For this review, take the finished solid that the model builds, in its own axes (mm). Face numbers are marked on the shaded views. A direction names the side the tool comes from. Give positions to 0.01 mm unless a question says otherwise; leave off trailing zeros. Loops run counter-clockwise (first coordinate to the right, second up) from the corner with the lowest first, then second, coordinate; pieces in that order, holes last.
Autodesk Inventor part; units mm, degrees
ref_plane "YZ Plane" through (0, 0, 0) normal (1, 0, 0) x (0, 1, 0)
ref_plane "XZ Plane" through (0, 0, 0) normal (0, 1, 0) x (-1, 0, 0)
ref_plane "XY Plane" through (0, 0, 0) normal (0, 0, 1) x (1, 0, 0)
sketch "Main Outline" plane through (0, 0, 0) normal (0, 0, 1) x (1, 0, 0)
  line L0 (0, 0) -> (304.8, 0) construction
  line L1 (304.8, 0) -> (304.8, 50.8) construction
  line L2 (304.8, 50.8) -> (0, 50.8) construction
  line L3 (0, 50.8) -> (0, 0) construction
  line L4 (0, 50.8) -> (0, 53.34) construction
  line L5 (0, 53.34) -> (304.8, 53.34) construction
  line L6 (304.8, 53.34) -> (304.8, 50.8) construction
  circle A0 centre (152.4, 23.8125) radius 17.4625 construction
  line L7 (152.4, 23.8125) -> (152.4, 0) construction
  circle A1 centre (152.4, 23.8125) radius 27.94 construction
  circle A2 centre (152.4, 23.8125) radius 21.59 construction
  line L8 (152.4, 23.8125) -> (144.1569, 60.2292) construction
  circle A3 centre (144.1569, 60.2292) radius 15.24 construction
  circle A4 centre (144.1569, 60.2292) radius 8.89 construction
  circle A5 centre (144.1569, 60.2292) radius 14.2875 construction
  arc A6 (163.8162, 72.0089) -> (128.198, 43.7805) centre (144.1569, 60.2292) ccw construction
  circle A7 centre (98.8106, 85.598) radius 32.258 construction
  circle A8 centre (124.5097, 147.0273) radius 32.258 construction
  circle A9 centre (174.158, 102.6533) radius 32.258 construction
  circle A10 centre (144.1569, 60.2292) radius 11.1125 construction
  circle A11 centre (152.4, 23.8125) radius 49.53 construction
  line L9 (144.1569, 60.2292) -> (124.5097, 147.0273) construction
  line L10 (144.1569, 60.2292) -> (98.8106, 85.598) construction
  line L11 (98.8106, 85.598) -> (174.158, 102.6533) construction
  line L12 (174.158, 102.6533) -> (144.1569, 60.2292) construction
  circle A12 centre (98.8106, 85.598) radius 9.5493 construction
  arc A13 (172.0498, 111.9669) -> (183.1109, 99.3313) centre (174.158, 102.6533) ccw construction
  circle A14 centre (124.5097, 147.0273) radius 9.5493 construction
  line L13 (96.7024, 94.9117) -> (172.0498, 111.9669) construction
  line L14 (183.1109, 99.3313) -> (165.6438, 52.2565) construction
  line L15 (92.161, 78.7444) -> (128.198, 43.7805) construction
  line L16 (172.0498, 111.9669) -> (174.158, 102.6533) construction
  line L17 (174.158, 102.6533) -> (183.1109, 99.3313) construction
  arc A15 (183.1109, 99.3313) -> (172.0498, 111.9669) centre (174.158, 102.6533) ccw construction
  arc A16 (165.6438, 52.2565) -> (163.8162, 72.0089) centre (144.1569, 60.2292) ccw construction
  arc A17 (128.198, 43.7805) -> (165.6438, 52.2565) centre (144.1569, 60.2292) ccw construction
  circle A18 centre (124.4396, 147.337) radius 32.258 construction
  circle A19 centre (124.3695, 147.6466) radius 32.258 construction
  circle A20 centre (124.2994, 147.9563) radius 32.258 construction
  line L18 (124.5097, 147.0273) -> (124.2994, 147.9563) construction
  circle A21 centre (124.5798, 146.7176) radius 32.258 construction
  circle A22 centre (117.4622, 43.2997) radius 9.525 construction
  circle A23 centre (175.54, 56.4459) radius 9.525 construction
  line L19 (152.4, 23.8125) -> (117.4622, 43.2997) construction
  line L20 (152.4, 23.8125) -> (175.54, 56.4459) construction
  line L21 (117.4622, 43.2997) -> (98.8106, 85.598) construction
  line L22 (175.54, 56.4459) -> (174.158, 102.6533) construction
  circle A24 centre (133.7342, 106.2753) radius 7.9375 construction
  line L23 (133.401, 150.5107) -> (165.496, 68.5894) construction
  circle A25 centre (152.4, 23.8125) radius 29.845 construction
  line L24 (114.985, 146.3422) -> (121.2977, 58.5849) construction
  circle A26 centre (99.0876, 85.443) radius 32.258 construction
  circle A27 centre (97.9793, 86.063) radius 32.258 construction
  line L25 (97.9793, 86.063) -> (98.8106, 85.598) construction
  circle A28 centre (98.2564, 85.908) radius 32.258 construction
  circle A29 centre (98.5335, 85.753) radius 32.258 construction
  circle A30 centre (152.4, 23.8125) radius 29.845 construction
  circle A31 centre (122.555, 23.8125) radius 6.35 construction
  circle A32 centre (179.3358, 36.6651) radius 6.35 construction
  line L26 (122.555, 23.8125) -> (152.4, 23.8125) construction
  line L27 (152.4, 23.8125) -> (182.245, 23.8125) construction
  circle A33 centre (182.245, 23.8125) radius 6.35 construction
  circle A34 centre (125.4642, 10.9599) radius 6.35 construction
  circle A35 centre (150.1885, 33.5827) radius 39.8623 construction
  line L28 (72.8944, 65.7819) -> (119.1902, 8.5205) construction
  circle A36 centre (174.708, 103.431) radius 32.258 construction
  line L29 (174.158, 102.6533) -> (174.708, 103.431) construction
  circle A37 centre (174.5246, 103.1717) radius 32.258 construction
  circle A38 centre (174.3413, 102.9125) radius 32.258 construction
  circle A39 centre (173.9747, 102.394) radius 32.258 construction
  line L30 (188.958, 24.3128) -> (206.0816, 95.9295) construction
  circle A40 centre (133.7342, 106.2753) radius 8.1693 construction
  arc A41 (85.4541, 115.7901) -> (94.2274, 135.7949) centre (79.2901, 130.4196) ccw construction
  arc A42 (156.6774, 149.9308) -> (173.2104, 135.6542) centre (172.4734, 151.5121) ccw construction
  line L31 (124.2994, 147.9563) -> (124.8602, 145.479) construction
  line L32 (114.3901, 145.7133) -> (114.9509, 143.236) construction
  line L33 (134.7695, 147.722) -> (134.2088, 150.1993) construction
  arc A43 (134.2088, 150.1993) -> (114.3901, 145.7133) centre (124.2994, 147.9563) ccw construction
  arc A44 (114.9509, 143.236) -> (134.7695, 147.722) centre (124.8602, 145.479) ccw construction
  line L34 (174.708, 103.431) -> (173.2414, 101.3571) construction
  line L35 (166.4126, 109.2972) -> (164.9461, 107.2234) construction
  line L36 (181.5368, 95.4909) -> (183.0033, 97.5647) construction
  arc A45 (183.0033, 97.5647) -> (166.4126, 109.2972) centre (174.708, 103.431) ccw construction
  arc A46 (164.9461, 107.2234) -> (181.5368, 95.4909) centre (173.2414, 101.3571) ccw construction
  line L37 (97.9793, 86.063) -> (100.196, 84.8229) construction
  line L38 (93.0188, 77.1963) -> (95.2355, 75.9562) construction
  line L39 (105.1564, 93.6897) -> (102.9398, 94.9298) construction
  arc A47 (102.9398, 94.9298) -> (93.0188, 77.1963) centre (97.9793, 86.063) ccw construction
  arc A48 (95.2355, 75.9562) -> (105.1564, 93.6897) centre (100.196, 84.8229) ccw construction
  circle A49 centre (117.4622, 43.2997) radius 3.9687 construction
  circle A50 centre (175.54, 56.4459) radius 3.9687 construction
  line L40 (152.4, 23.8125) -> (158.9889, -5.2961) construction
  arc A51 (89.3511, 54.6895) -> (85.9237, 49.6664) centre (88.3927, 51.6626) ccw construction
  arc A52 (201.2624, 75.7739) -> (196.006, 78.8314) centre (198.1744, 76.5122) ccw construction
  circle A53 centre (152.4, 23.8125) radius 14.224 construction
  circle A54 centre (133.7342, 106.2753) radius 3.9687 construction
  circle A55 centre (156.886, 3.9939) radius 6.35 construction
  circle A56 centre (156.886, 3.9939) radius 2.0828 construction
  circle A57 centre (152.4, 23.8125) radius 20.32 construction
  line L41 (132.9935, 29.8368) -> (152.4, 23.8125) construction
  line L42 (152.4, 23.8125) -> (167.3204, 37.6068) construction
  circle A58 centre (167.3204, 37.6068) radius 2.0828 construction
  circle A59 centre (167.3204, 37.6068) radius 3.9687 construction
  circle A60 centre (132.9935, 29.8368) radius 2.0828 construction
  circle A61 centre (132.9935, 29.8368) radius 3.9688 construction
  point P0 (173.9747, 102.394)
  point P1 (99.0876, 85.443)
  dimension "d18" = 99.06
  dimension "d58" = 64.516
  dimension "d86" = 64.516
  dimension "d0" = 304.8
  dimension "d1" = 50.8
  dimension "d2" = 2.54
  dimension "d3" = 34.925
  dimension "d4" = 23.8125
  dimension "d5" = 152.4
  dimension "d6" = 55.88
  dimension "d7" = 43.18
  dimension "d8" = 37.338
  dimension "d10" = 30.48
  dimension "d11" = 17.78
  dimension "d12" = 28.575
  dimension "d13" = 45.8366
  dimension "d14" = 64.516
  dimension "d15" = 64.516
  dimension "d16" = 64.516
  dimension "d17" = 22.225
  dimension "d19" = 51.9602
  dimension "d20" = 88.9939
  dimension "d21" = 19.0986
  dimension "d22" = 19.0986
  dimension "d23" = 19.0986
  dimension "d30" = 123.112
  dimension "d40" = 64.516
  dimension "d41" = 64.516
  dimension "d42" = 64.516
  dimension "d43" = 0.9525
  dimension "d44" = 0.3175
  dimension "d45" = 0.635
  dimension "d46" = 64.516
  dimension "d47" = 0.3175
  dimension "d48" = 19.05
  dimension "d49" = 19.05
  dimension "d50" = 40.005
  dimension "d51" = 40.005
  dimension "d52" = 46.228
  dimension "d54" = 46.228
  dimension "d55" = 15.875
  dimension "d56" = 41.4655
  dimension "d57" = 59.69
  dimension "d59" = 64.516
  dimension "d60" = 64.516
  dimension "d61" = 64.516
  dimension "d62" = 0.3175
  dimension "d63" = 0.3175
  dimension "d64" = 0.635
  dimension "d65" = 0.9525
  dimension "d73" = 12.7
  dimension "d74" = 12.7
  dimension "d76" = 59.69
  dimension "d78" = 12.7
  dimension "d79" = 12.7
  dimension "d80" = 64.516
  dimension "d81" = 0.9525
  dimension "d82" = 64.516
  dimension "d83" = 64.516
  dimension "d84" = 0.3175
  dimension "d85" = 0.635
  dimension "d88" = 0.3175
  dimension "d89" = 31.75
  dimension "d90" = 31.75
  dimension "d94" = 1.5875
  dimension "d95" = 20.32
  dimension "d96" = 1.5875
sketch "Upper CIM C-C Check" plane through (0, 0, 0) normal (0, 0, 1) x (1, 0, 0)
  arc A0 (3.4429, -22.6582) -> (3.4429, 22.6582) centre (0, 0) ccw construction
  arc A1 (90.4285, 9.4409) -> (90.4285, -9.4409) centre (88.9939, 0) ccw construction
  line L0 (88.9939, 0) -> (0, 0) construction
  line L1 (90.4285, 9.4409) -> (3.4429, 22.6582)
  line L2 (3.4429, -22.6582) -> (90.4285, -9.4409)
  arc A2 (90.4285, -9.4409) -> (90.4285, 9.4409) centre (88.9939, 0) ccw
  arc A3 (3.4429, 22.6582) -> (3.4429, -22.6582) centre (0, 0) ccw
  dimension "d24" = 45.8366
  dimension "d25" = 19.0986
  dimension "d26" = 78.9119
  dimension "d27" = 87.984
  dimension "d28" = 27.12
  dimension "d29" = 88.9939
sketch "Sketch3" plane through (0, 0, 0) normal (1, 0, 0) x (0, 1, 0)
  line L0 (0, 0) -> (50.8, 0)
  line L1 (50.8, 0) -> (50.8, -50.8)
  line L2 (50.8, -50.8) -> (0, -50.8)
  line L3 (0, -50.8) -> (0, 0)
  line L4 (3.175, -3.175) -> (47.625, -3.175)
  line L5 (47.625, -3.175) -> (47.625, -47.625)
  line L6 (47.625, -47.625) -> (3.175, -47.625)
  line L7 (3.175, -47.625) -> (3.175, -3.175)
  dimension "d115" = 50.8
  dimension "d116" = 50.8
  dimension "d117" = 44.45
  dimension "d118" = 44.45
  dimension "d119" = 3.175
  dimension "d120" = 3.175
extrude "Extrusion1" add sketch "Sketch3" along normal blind 304.8
sketch "Sketch4" plane through (0, 0, 0) normal (0, 0, 1) x (1, 0, 0)
  circle A0 centre (152.4, 23.8125) radius 9.525
  circle A1 centre (117.4622, 43.2997) radius 4.7625
  circle A2 centre (144.1569, 60.2292) radius 12.7
  point P0 (0, 0)
  point P1 (122.555, 23.8125)
  point P2 (125.4642, 10.9599)
  point P3 (182.245, 23.8125)
  point P4 (179.3358, 36.6651)
  dimension "d123" = 19.05
  dimension "d124" = 9.525
  dimension "d134" = 25.4
extrude "Extrusion2" cut sketch "Sketch4" against normal up to surface (3.175 mm away) contours A0 | A1
hole "Hole1" at (122.555, 23.8125, 0) at (182.245, 23.8125, 0) direction (0, 0, -1) diameter 6.5278 end up to surface
extrude "Extrusion3" cut sketch "Sketch4" against normal up to surface (50.8 mm away) contours A2
fillet "Fillet1" radius 25.4 2 edges at (135.6493, 50.8, -25.4) (152.6645, 50.8, -25.4)
equation "\"d3\" = r10"
equation "\"d6\" = g44"
equation "\"d7\" = g34"
equation "\"d10\" = g24"
equation "\"d11\" = g14"
equation "\"d12\" = r8"
equation "\"d13\" = p48"
equation "\"d14\" = cim"
equation "\"d15\" = cim"
equation "\"d16\" = cim"
equation "\"d17\" = r6"
equation "\"d21\" = p20"
equation "\"d22\" = p20"
equation "\"d23\" = p20"
equation "\"d24\" = p48"
equation "\"d25\" = p20"
equation "\"d29\" = d20"
equation "\"g14\" = 17.78"
equation "\"g24\" = 30.48"
equation "\"g34\" = 43.18"
equation "\"g44\" = 55.88"
equation "\"p20\" = 19.09859"
equation "\"p48\" = 45.83662"
equation "\"r10\" = 34.925"
equation "\"r9\" = 31.75"
equation "\"r8\" = 28.575"
equation "\"r7\" = 25.4"
equation "\"r6\" = 22.225"
equation "\"r5\" = 19.05"
equation "\"r4\" = 15.875"
equation "\"r3\" = 12.7"
equation "\"cim\" = 64.516"
equation "\"act\" = 28.448"
equation "\"actL\" = 23.749"
equation "\"UpperCimCCCheck\" = 2 * d27 + d26 + d28"
equation "\"LowerBeltPathCCCheck\" = 267"
properties material "Aluminum 6061"
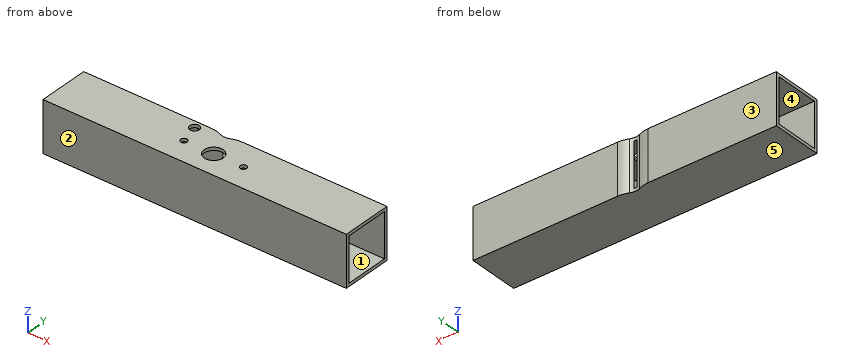
Item 1: Take a section at C-C on y = 11. Give the boundary of the cut face in (x, z) (3 decimals).
Answer:
outline: (0, -50.8) - (304.8, -50.8) - (304.8, -47.625) - (0, -47.625) - close; (0, -3.175) - (304.8, -3.175) - (304.8, 0) - (0, 0) - close
Item 2: Take a section at B-B on z = -33.5. Give the boundary of the cut face in (x, y) (3 decimals).
Answer:
outline: (0, 0) - (304.8, 0) - (304.8, 3.175) - (0, 3.175) - close; (0, 47.625) - (142.6, 47.625) arc R12.7 cw to (139.009, 48.619) arc R25.4 ccw to (128.712, 50.8) - (0, 50.8) - close; (145.714, 47.625) - (304.8, 47.625) - (304.8, 50.8) - (159.602, 50.8) arc R25.4 ccw to (149.305, 48.619) arc R12.7 cw to start
Item 3: For L1, parallel to Z at x = 187, y = 42 (3 decimals); L2, parallel to Y at x = 178, z = -25 (3 decimals); L3, parallel to Y at x = 155, z = -25 (3 decimals), list the stretches that pass through material, from the lowest coordinate up.
Answer:
L1: z = -50.8 to -47.625, -3.175 to 0
L2: y = 0 to 3.175, 47.625 to 50.8
L3: y = 0 to 3.175, 47.625 to 50.38
Item 4: Clearance check with flat-ended pins moving along their axes: pin 1 Ø5 at (y, z) = (44.5, -16.5) entering from +X; pin 2 Ø6 at (x, z) = (154, -35) entering from +Y; pin 3 Ø5 at (x, y) = (122.56, 23.81) entering from +Z (3 decimals). State where each tip first meets the part, or that it passes through.
Answer:
pin 1: passes through
pin 2: stops at y = 50.67
pin 3: stops at z = -47.625
Item 5: Take a section at D-D on x = 152.4. Give the boundary of the cut face in (y, z) (1 decimal), and give its area (3 significant figures).
Answer:
outline: (0, -50.8) - (49.8, -50.8) - (49.8, 0) - (33.3, 0) - (33.3, -3.2) - (47.6, -3.2) - (47.6, -47.6) - (3.2, -47.6) - (3.2, -3.2) - (14.3, -3.2) - (14.3, 0) - (0, 0) - close
area: 491 mm2
Item 6: The part is to be moulded in two halves that separate along Y. For the marked faces 3, 4 and 5, say which applies: released by +Y, released by -Y, zero draft, split by the parting line, or undercut.
Answer:
face 3: released by +Y
face 4: undercut
face 5: zero draft
Item 7: Take a section at A-A on x = 191.5. Give the boundary of the cut face in (y, z) (3 decimals).
Answer:
outline: (0, -50.8) - (50.8, -50.8) - (50.8, 0) - (0, 0) - close; hole (3.175, -47.625) - (47.625, -47.625) - (47.625, -3.175) - (3.175, -3.175) - close
Item 8: Tool access review of the marked faces 1 and 2: name each direction out of +Z, -Z, +X, -X, +Y, -Y from which nothing blocks a thin tool from reaching the whole face with its end or side.
Answer:
face 1: +X, -X
face 2: +Z, -Z, +X, -X, -Y
